Part model, mm, in its own coordinate system. Face numbers are marked on the shaded views. Coordinates: 2 decimals unless noted, no trailing zeros. Loops run counter-clockwise (first coordinate to the right, second up) from the corner with the lowest first, then second, coordinate; pieces in that order, holes last. Notation, with made-up numbers: M -3,-32.5 L 45,-32.5 A15 ccw 45,-4.5 Z; hole C 18,73 d1. An arc over 180 degrees is marked long. Use a Markdown table: item, result. Add a question column.
1) Pull direction X, two halves, no side cores. Call the marked faces 1, 2 and 3: released by +X, released by -X, zero draft, split by the parting line, or undercut.
2) Band-saw the part on A-A (y = 168.5). List the corners of the cut face in (x, z) (3 decimals).
3) Wall check: probe 1 along Z at (x, y) = (-231, 178); probe 2 along X at (y, z) = (0.6, 20); probe 3 along X at (y, z) = (1, 20). Give the ranges that are in metal, low to high. Write a range as from..to.
4) Band-saw the part on B-B (z = 32). List the corners of the cut face in (x, y) (3 decimals).
5) Band-saw the part on D-D (x = -65). List the corners of the cut face in (y, z) (3 decimals).
6) Pin check, flat tips, straight feed: pin 1 Ø6.5 at (x, z) = (19.05, 20) entering from -Y; pin 2 Ø12 at (x, z) = (26, 20) entering from +Y (3 decimals); pin 3 Ø4 at (y, z) = (93, 6.5) entering from -X; pin 4 Ø12 at (x, z) = (-85.5, 25.5) entering from +Y. Stop position of each tip, or through.
7) Band-saw the part on C-C (y = 32). List the corners of the cut face in (x, z).
from build123d import *

# Parameters (mm, degrees)
BOSS_EXTRUDE1_DEPTH     = 40
CUT_EXTRUDE1_DEPTH      = 306.96246604
CUT_EXTRUDE1_DEPTH_BACK = 306.96246604
SKETCH3_R               = 2.5
CUT_EXTRUDE2_DEPTH      = 507.98027575
CUT_EXTRUDE2_DEPTH_BACK = 507.98027575
SKETCH4_R               = 1.984375


with BuildPart() as part:
    # Sketch1 → Boss-Extrude1 (new body)
    with BuildSketch(Plane.XY):
        Polygon((-80, 0), (80, 0), (232.5, 148), (232.5, 198), (229.325, 198), (229.325, 149.343064798), (78.712635935, 3.175), (-78.712635935, 3.175), (-229.325, 149.343064798), (-229.325, 198), (-232.5, 198), (-232.5, 148), align=None)
    extrude(amount=BOSS_EXTRUDE1_DEPTH)

    # Sketch3 → Cut-Extrude1 (cut, two sides: drawn at the far end of the back side and taken through both)
    with BuildSketch(Plane(origin=(0, 3.175, 0), x_dir=(1, 0, 0), z_dir=(0, 1, 0)).offset(-CUT_EXTRUDE1_DEPTH_BACK)):
        with Locations(Location((-19.05, -20, 0), (0, 0, 270))):
            Circle(SKETCH3_R)
        with Locations(Location((19.05, -20, 0), (0, 0, 270))):
            Circle(SKETCH3_R)
    extrude(amount=CUT_EXTRUDE1_DEPTH + CUT_EXTRUDE1_DEPTH_BACK, mode=Mode.SUBTRACT)

    # Sketch4 → Cut-Extrude2 (cut, two sides: drawn at the far end of the back side and taken through both)
    with BuildSketch(Plane.ZY.offset(232.5).offset(-CUT_EXTRUDE2_DEPTH_BACK)):
        with Locations((20, 178)):
            Circle(SKETCH4_R)
    extrude(amount=CUT_EXTRUDE2_DEPTH + CUT_EXTRUDE2_DEPTH_BACK, mode=Mode.SUBTRACT)


solid = part.part
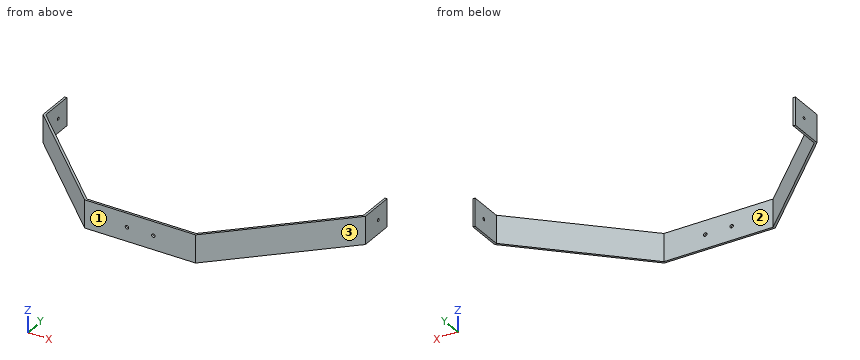
Entries:
| question | item | result |
|---|---|---|
| 1 | face 1 | zero draft |
| 1 | face 2 | undercut |
| 1 | face 3 | released by +X |
| 2 | outline | M -232.5,0 L -229.325,0 L -229.325,40 L -232.5,40 Z; M 229.325,0 L 232.5,0 L 232.5,40 L 229.325,40 Z |
| 3 | probe 1 | 0..18.02, 21.98..40 |
| 3 | probe 2 | -80.62..-21.55, -16.55..16.55, 21.55..80.62 |
| 3 | probe 3 | -81.03..-21.55, -16.55..16.55, 21.55..81.03 |
| 4 | outline | M -232.5,148 L -80,0 L 80,0 L 232.5,148 L 232.5,198 L 229.325,198 L 229.325,149.343 L 78.713,3.175 L -78.713,3.175 L -229.325,149.343 L -229.325,198 L -232.5,198 Z |
| 5 | outline | M 0,0 L 3.175,0 L 3.175,40 L 0,40 Z |
| 6 | pin 1 | y = 0 |
| 6 | pin 2 | y = 3.175 |
| 6 | pin 3 | x = -177.89 |
| 6 | pin 4 | y = 15.59 |
| 7 | outline | M -112.97,0 L -108.41,0 L -108.41,40 L -112.97,40 Z; M 108.41,0 L 112.97,0 L 112.97,40 L 108.41,40 Z |
